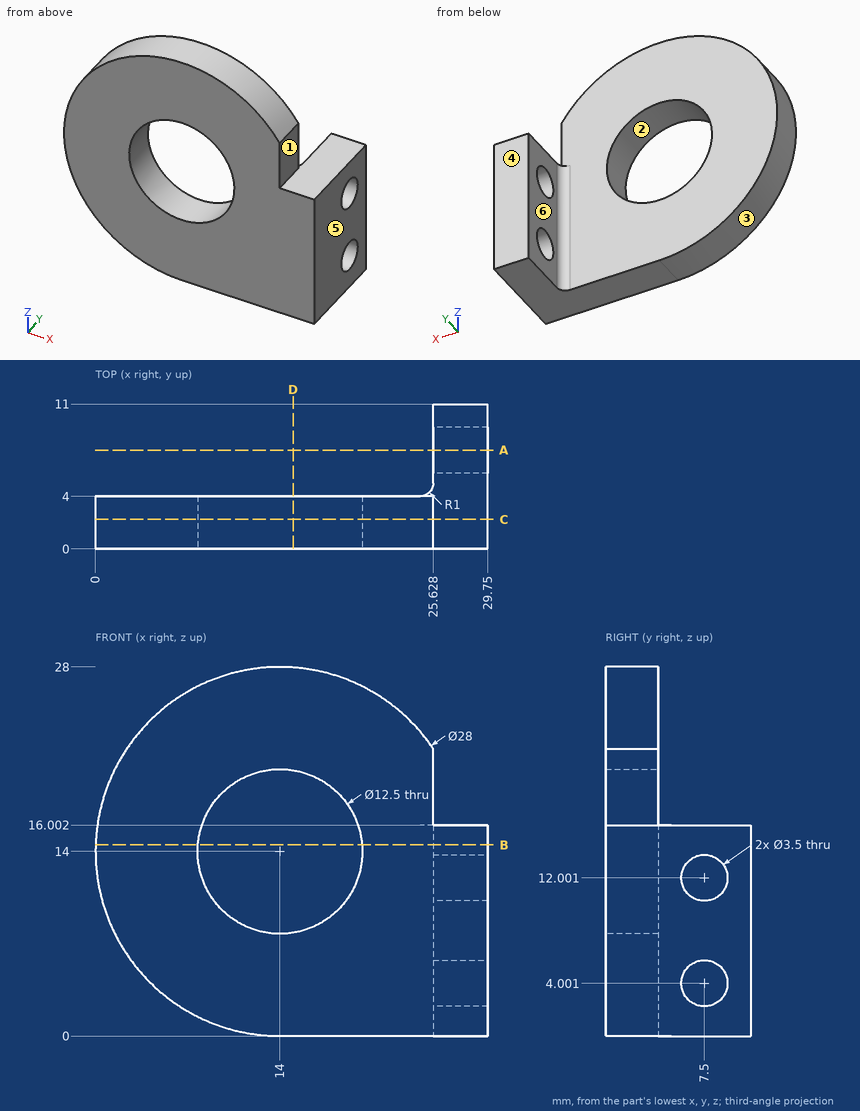
Here's the drawing with two shaded views (mm, measured from the low corner). I have some questions. A direction names the side the tool comes from. Coordinates: 2 decimals unless noted, no trailing zeros. Write each loop counter-clockwise with the first axis right and the second up, starting at its lowest first coordinate (ties: lowest second). Pieces come first, ordered by that corner, then holes. Notation, with made-up numbers: (-36, -1) -> (12, -1) arc R28 cw to (12, 22) -> close; hole circle Ø4 at (24.25, 80.25). An arc over 180 degrees is marked (long way). Answer as CSV lines item,"result".
1) On a 3-axis mill with a long thin cutter (end or side, diameter ignored), from which of +Z, -Z, +X, -X, +Y, -Y can I reach the whole of each face in a straight line? I mean the marked faces 5 and 6. Say none if no direction works.
Check result:
face 5,"+Z, -Z, +X, +Y, -Y"
face 6,"+Z, -Z, -X, +Y"
2) If we section it at A-A on y = 7.5: Please give me the cut outline in (x, z).
Check result:
outline,"(25.63, 0) -> (29.75, 0) -> (29.75, 2.25) -> (25.63, 2.25) -> close; (25.63, 5.75) -> (29.75, 5.75) -> (29.75, 10.25) -> (25.63, 10.25) -> close; (25.63, 13.75) -> (29.75, 13.75) -> (29.75, 16) -> (25.63, 16) -> close"
3) If we section it at B-B on z = 14.5: Please give me the cut outline in (x, y).
Check result:
outline,"(0.01, 0) -> (7.77, 0) -> (7.77, 4) -> (0.01, 4) -> close; (20.23, 0) -> (29.75, 0) -> (29.75, 11) -> (25.63, 11) -> (25.63, 5) arc R1 cw to (24.63, 4) -> (20.23, 4) -> close"
4) If we section it at D-D on x = 15: Please give me the cut outline in (y, z) (1 decimal).
Check result:
outline,"(0, 0) -> (4, 0) -> (4, 7.8) -> (0, 7.8) -> close; (0, 20.2) -> (4, 20.2) -> (4, 28) -> (0, 28) -> close"
5) If I drill on line 1 (X direction, y = 3.2, z = 14); line 2 (Y direction, x = 22.25, z = 3.5); line 3 (X direction, y = 10, z = 13.75), over which ranges is the centre line in solid material (lowest first)? Write a range as from..to.
Check result:
line 1,"0..7.75, 20.25..29.75"
line 2,"0..4"
line 3,"25.63..29.75"
6) If we section it at C-C on y = 2.25: Please give me the cut outline in (x, z), then the cut area to 3 significant figures.
Check result:
outline,"(14, 0) -> (29.75, 0) -> (29.75, 16) -> (25.63, 16) -> (25.63, 21.8) arc R14 ccw (long way) to start; hole circle Ø12.5 at (14, 14)"
area,"555 mm²"
7) Will these pins go through, and if not, where does the flat tip stop? P1, Ø2, axis at y = 7.5, z = 4, coming from the +X side; P2, Ø3, axis at x = 7, y = 2, coming from the +Z side (1 decimal); P3, Ø1.5, axis at y = 6.5, z = 9, coming from the -X side; P4, Ø4.5, axis at y = 2, z = 20, coming from the +X side.
Check result:
P1,"through"
P2,"z = 26.9"
P3,"x = 25.63"
P4,"x = 25.63"
8) If we mould it in two halves opening along X, with no side actions, what happens to the marked faces 1, 2, 3 and 4? For each: +X half, -X half, draft (parallel to the pull), parting line (faces both ways), or undercut.
Check result:
face 1,"+X half"
face 2,"undercut"
face 3,"parting line"
face 4,"draft"
